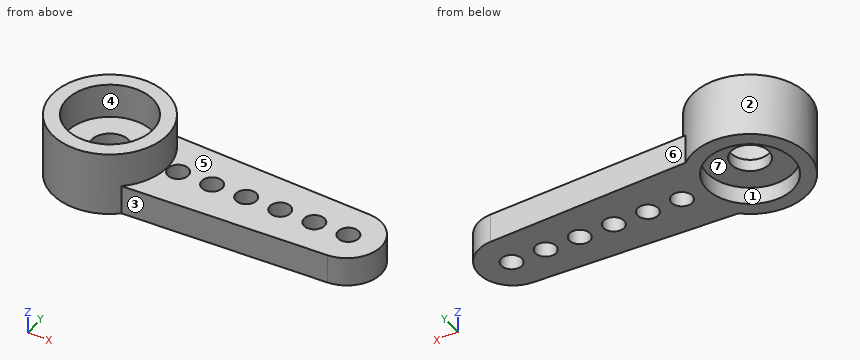
```python
from build123d import *

# Parameters (mm, degrees)
F0_R     = 0.6
F1_DEPTH = 1.7
F2_R     = 3.35
F3_DEPTH = 2
F4_R     = 2.5
F5_DEPTH = 1
F6_R     = 1.1
F7_DEPTH = 2.701
F8_R     = 2.5
F9_DEPTH = 2


with BuildPart() as f1:
    # F0 (on Top) → F1 (new body)
    with BuildSketch(Plane.XY):
        with BuildLine():
            ThreePointArc((2.2299103121, -2.5), (3.057180036, -1.369726333), (3.35, 0))
            ThreePointArc((3.35, 0), (3.057180036, 1.369726333), (2.2299103121, 2.5))
            ThreePointArc((2.2299103121, 2.5), (-3.35, 0), (2.2299103121, -2.5))
        make_face()
        with BuildLine():
            ThreePointArc((2.2299103121, 2.5), (3.057180036, 1.369726333), (3.35, 0))
            ThreePointArc((3.35, 0), (3.057180036, -1.369726333), (2.2299103121, -2.5))
            Line((2.2299103121, -2.5), (14, -2))
            ThreePointArc((14, -2), (15.9168426648, 0), (14, 2))
            Line((14, 2), (2.2299103121, 2.5))
        make_face()
        with Locations((4, 0)):
            Circle(F0_R, mode=Mode.SUBTRACT)
        with Locations((6, 0)):
            Circle(F0_R, mode=Mode.SUBTRACT)
        with Locations((8, 0)):
            Circle(F0_R, mode=Mode.SUBTRACT)
        with Locations((10, 0)):
            Circle(F0_R, mode=Mode.SUBTRACT)
        with Locations((12, 0)):
            Circle(F0_R, mode=Mode.SUBTRACT)
        with Locations((14, 0)):
            Circle(F0_R, mode=Mode.SUBTRACT)
    extrude(amount=F1_DEPTH)

    # F2 (on face) → F3 (join)
    with BuildSketch(Plane.XY.offset(1.7)):
        Circle(F2_R)
    extrude(amount=F3_DEPTH)

    # F4 (on face) → F5 (cut)
    with BuildSketch(Plane(origin=(0, 0, 0), x_dir=(1, 0, 0), z_dir=(0, 0, -1))):
        Circle(F4_R)
    extrude(amount=-F5_DEPTH, mode=Mode.SUBTRACT)

    # F6 (on face) → F7 (cut, through all)
    with BuildSketch(Plane(origin=(0, 0, 1), x_dir=(1, 0, 0), z_dir=(0, 0, -1))):
        Circle(F6_R)
    extrude(amount=-F7_DEPTH, mode=Mode.SUBTRACT)

    # F8 (on face) → F9 (cut)
    with BuildSketch(Plane.XY.offset(3.7)):
        Circle(F8_R)
    extrude(amount=-F9_DEPTH, mode=Mode.SUBTRACT)


solid = f1.part
```
Read the model definition and answer for the solid it produces. Units are mm, in the model's axes. Face numbers are marked on the shaded views. A direction names the side the tool comes from. Give positions to 0.01 mm unless a question says otherwise; leave off trailing zeros. Loops run counter-clockwise (first coordinate to the right, second up) from the corner with the lowest first, then second, coordinate; pieces in that order, holes last.
Item 1: The part is cut by section C-C (y = 0). Give the number of separate pieces and of enclosed holes in the cut face, and give its area (3 significant figures).
Item 2: The part is cut by section B-B (x = 0). Write down the section's boundary in (y, z).
Item 3: The part is cut by section A-A (z = 0.45). Write down the section's boundary in (x, y), and give its area (3 significant figures).
Item 4: Find the intervals of material crossed by line 1 along Y through (x, z) = (14, 1.45); line 2 along Z through (x, y) = (9.75, 1); line 3 along Y through (x, z) = (12, 0.3), in increasing order.
Item 5: The mould has two halves that part along Y. Classify the marked faces 4, 5, 6 and 7: released by +Y, released by -Y, zero draft, split by the parting line, or undercut.
Item 6: The part is cut by section D-D (x = 6). Write down the section's boundary in (y, z).
Item 7: For the marked faces 1, 2 and 3, determine the directions among +Z, -Z, +X, -X, +Y, -Y from which every point of the face is accessible in a straight line to the end or side of a thin tool.
Item 8: Each of these flat-tipped pins is pushed along its axis until it touches: pin 1 Ø2 at (x, z) = (6, 2.5) entering from -Y; pin 2 Ø1.4 at (x, y) = (10, 0) entering from +Z; pin 3 Ø3 at (x, y) = (0, 0) entering from -Z. Where does it stop, or does it pass through?
Taken from the geometry:
1. separate pieces: 8
1. enclosed holes: 0
1. area: 17.4 mm2
2. outline: (-3.35, 0) - (-2.5, 0) - (-2.5, 1) - (-1.1, 1) - (-1.1, 1.7) - (-2.5, 1.7) - (-2.5, 3.7) - (-3.35, 3.7) - close; (1.1, 1) - (2.5, 1) - (2.5, 0) - (3.35, 0) - (3.35, 3.7) - (2.5, 3.7) - (2.5, 1.7) - (1.1, 1.7) - close
3. outline: (2.23, -2.5) - (14, -2) arc R2 ccw to (14, 2) - (2.23, 2.5) arc R3.35 ccw (long way) to start; hole circle Ø5 at (0, 0); hole circle Ø1.2 at (4, 0); hole circle Ø1.2 at (6, 0); hole circle Ø1.2 at (8, 0); hole circle Ø1.2 at (10, 0); hole circle Ø1.2 at (12, 0); hole circle Ø1.2 at (14, 0)
3. area: 63.9 mm2
4. line 1: y = -2 to -0.6, 0.6 to 2
4. line 2: z = 0 to 1.7
4. line 3: y = -2.08 to -0.6, 0.6 to 2.08
5. face 4: undercut
5. face 5: zero draft
5. face 6: released by +Y
5. face 7: undercut
6. outline: (-2.34, 0) - (-0.6, 0) - (-0.6, 1.7) - (-2.34, 1.7) - close; (0.6, 0) - (2.34, 0) - (2.34, 1.7) - (0.6, 1.7) - close
7. face 1: -Z
7. face 2: +Z
7. face 3: +Z, -Z, +X, -Y
8. pin 1: stops at y = -2.37
8. pin 2: stops at z = 1.7
8. pin 3: stops at z = 1
